Work out the finished part from the listing and answer in its coordinate system (mm). A direction names the side the tool comes from. Coordinates: 2 decimals unless noted, no trailing zeros. Loops run counter-clockwise (first coordinate to the right, second up) from the corner with the lowest first, then second, coordinate; pieces in that order, holes last. Notation, with made-up numbers: (0, 15.5) -> (26, 15.5) arc R7 cw to (26, 23.5) -> close; hole circle Ø4 at (67.5, 63.25). An arc over 180 degrees is marked (long way). Answer as CSV lines item,"result".
```python
from build123d import *

# Parameters (mm, degrees)
PAD_DEPTH         = 2
PAD001_DEPTH      = 4
PAD002_DEPTH      = 8
SKETCH002_R       = 2.5
PAD003_DEPTH      = 22.4
CYLINDER_R        = 6
CYLINDER_DEPTH    = 4
CYLINDER001_R     = 6
CYLINDER001_DEPTH = 4
CYLINDER002_R     = 6
CYLINDER002_DEPTH = 4
CYLINDER003_R     = 6
CYLINDER003_DEPTH = 4
CYLINDER004_R     = 3
CYLINDER004_DEPTH = 2
CYLINDER005_R     = 3
CYLINDER005_DEPTH = 2
CYLINDER006_R     = 3
CYLINDER006_DEPTH = 2
CYLINDER007_R     = 3
CYLINDER007_DEPTH = 2
SKETCH003_R       = 1.65
POCKET_DEPTH      = 22.4


with BuildPart() as part:
    # Sketch004 → Pad (new body)
    with BuildSketch(Plane.XY):
        with BuildLine():
            Line((74.149994, 7), (74.149994, 114.650046))
            ThreePointArc((74.149994, 114.650046), (72.099741, 119.599793), (67.149994, 121.650046))
            Line((67.149994, 121.650046), (7, 121.650046))
            ThreePointArc((7, 121.650046), (2.050253, 119.599793), (0, 114.650046))
            Line((0, 114.650046), (0, 7))
            ThreePointArc((0, 7), (2.050253, 2.050253), (7, 0))
            Line((7, 0), (67.149994, 0))
            ThreePointArc((67.149994, 0), (72.099741, 2.050253), (74.149994, 7))
        make_face()
    extrude(amount=PAD_DEPTH)

    # Sketch001 → Pad001 (join)
    with BuildSketch(Plane.XY):
        with BuildLine():
            Line((74.149994, 7), (74.149994, 114.650046))
            ThreePointArc((74.149994, 114.650046), (72.099741, 119.599793), (67.149994, 121.650046))
            Line((67.149994, 121.650046), (7, 121.650046))
            ThreePointArc((7, 121.650046), (2.050253, 119.599793), (0, 114.650046))
            Line((0, 114.650046), (0, 7))
            ThreePointArc((0, 7), (2.050253, 2.050253), (7, 0))
            Line((7, 0), (67.149994, 0))
            ThreePointArc((67.149994, 0), (72.099741, 2.050253), (74.149994, 7))
        make_face()
        with BuildLine():
            Line((7, 3), (67.149994, 3))
            ThreePointArc((67.149994, 3), (69.978421, 4.171573), (71.149994, 7))
            Line((71.149994, 7), (71.149994, 114.650046))
            ThreePointArc((71.149994, 114.650046), (69.978421, 117.478473), (67.149994, 118.650046))
            Line((67.149994, 118.650046), (7, 118.650046))
            ThreePointArc((7, 118.650046), (4.171573, 117.478473), (3, 114.650046))
            Line((3, 114.650046), (3, 7))
            ThreePointArc((3, 7), (4.171573, 4.171573), (7, 3))
        make_face(mode=Mode.SUBTRACT)
    extrude(amount=PAD001_DEPTH)

    # Sketch → Pad002 (join)
    with BuildSketch(Plane.XY):
        with BuildLine():
            Line((74.149994, 7), (74.149994, 114.650046))
            ThreePointArc((74.149994, 114.650046), (72.099741, 119.599793), (67.149994, 121.650046))
            Line((67.149994, 121.650046), (7, 121.650046))
            ThreePointArc((7, 121.650046), (2.050253, 119.599793), (0, 114.650046))
            Line((0, 114.650046), (0, 7))
            ThreePointArc((0, 7), (2.050253, 2.050253), (7, 0))
            Line((7, 0), (67.149994, 0))
            ThreePointArc((67.149994, 0), (72.099741, 2.050253), (74.149994, 7))
        make_face()
        with BuildLine():
            Line((7, 1.4), (67.149994, 1.4))
            ThreePointArc((67.149994, 1.4), (71.109792, 3.040202), (72.749994, 7))
            Line((72.749994, 7), (72.749994, 114.650046))
            ThreePointArc((72.749994, 114.650046), (71.109792, 118.609844), (67.149994, 120.250046))
            Line((67.149994, 120.250046), (7, 120.250046))
            ThreePointArc((7, 120.250046), (3.040202, 118.609844), (1.4, 114.650046))
            Line((1.4, 114.650046), (1.4, 7))
            ThreePointArc((1.4, 7), (3.040202, 3.040202), (7, 1.4))
        make_face(mode=Mode.SUBTRACT)
    extrude(amount=PAD002_DEPTH)

    # Sketch002 → Pad003 (join)
    with BuildSketch(Plane.XY):
        with Locations((12.075062, 22.075062)):
            Circle(SKETCH002_R)
        with Locations((12.075024, 109.57503)):
            Circle(SKETCH002_R)
        with Locations((62.075044, 109.575056)):
            Circle(SKETCH002_R)
        with Locations((62.075039, 22.075116)):
            Circle(SKETCH002_R)
    extrude(amount=PAD003_DEPTH)

    # Cylinder → Cylinder (join)
    with BuildSketch(Plane(origin=(12.075062, 22.075062, 0), x_dir=(0, -1, 0), z_dir=(0, 0, 1))):
        Circle(CYLINDER_R)
    extrude(amount=CYLINDER_DEPTH)

    # Cylinder001 → Cylinder001 (join)
    with BuildSketch(Plane(origin=(62.075039, 22.075116, 0), x_dir=(0, -1, 0), z_dir=(0, 0, 1))):
        Circle(CYLINDER001_R)
    extrude(amount=CYLINDER001_DEPTH)

    # Cylinder002 → Cylinder002 (join)
    with BuildSketch(Plane(origin=(62.075044, 109.575056, 0), x_dir=(0, -1, 0), z_dir=(0, 0, 1))):
        Circle(CYLINDER002_R)
    extrude(amount=CYLINDER002_DEPTH)

    # Cylinder003 → Cylinder003 (join)
    with BuildSketch(Plane(origin=(12.075024, 109.57503, 0), x_dir=(0, -1, 0), z_dir=(0, 0, 1))):
        Circle(CYLINDER003_R)
    extrude(amount=CYLINDER003_DEPTH)

    # Cylinder004 → Cylinder004 (cut)
    with BuildSketch(Plane(origin=(12.075062, 22.075062, 0), x_dir=(0, -1, 0), z_dir=(0, 0, 1))):
        Circle(CYLINDER004_R)
    extrude(amount=CYLINDER004_DEPTH, mode=Mode.SUBTRACT)

    # Cylinder005 → Cylinder005 (cut)
    with BuildSketch(Plane(origin=(62.075039, 22.075116, 0), x_dir=(0, -1, 0), z_dir=(0, 0, 1))):
        Circle(CYLINDER005_R)
    extrude(amount=CYLINDER005_DEPTH, mode=Mode.SUBTRACT)

    # Cylinder006 → Cylinder006 (cut)
    with BuildSketch(Plane(origin=(12.075024, 109.57503, 0), x_dir=(0, -1, 0), z_dir=(0, 0, 1))):
        Circle(CYLINDER006_R)
    extrude(amount=CYLINDER006_DEPTH, mode=Mode.SUBTRACT)

    # Cylinder007 → Cylinder007 (cut)
    with BuildSketch(Plane(origin=(62.075044, 109.575056, 0), x_dir=(0, -1, 0), z_dir=(0, 0, 1))):
        Circle(CYLINDER007_R)
    extrude(amount=CYLINDER007_DEPTH, mode=Mode.SUBTRACT)

    # Sketch003 → Pocket (cut)
    with BuildSketch(Plane.XY):
        with Locations((12.075062, 22.075062)):
            Circle(SKETCH003_R)
        with Locations((12.075024, 109.57503)):
            Circle(SKETCH003_R)
        with Locations((62.075044, 109.575056)):
            Circle(SKETCH003_R)
        with Locations((62.075039, 22.075116)):
            Circle(SKETCH003_R)
    extrude(amount=POCKET_DEPTH, mode=Mode.SUBTRACT)


solid = part.part
```
(1) Flat-ended cylindrical pins translate along their axes: pin 1 Ø5 at (x, y) = (13, 21) entering from -Z; pin 2 Ø6 at (x, z) = (17, 18.5) entering from -Y; pin 3 Ø10 at (x, z) = (45.5, 17) entering from +Y; pin 4 Ø6 at (x, y) = (14, 79.5) entering from +Z. Find the tip coordinate at first contact, or state that the pin passes through.
Computed values:
pin 1,"z = 0"
pin 2,"y = 20.48"
pin 3,"through"
pin 4,"z = 2"
(2) A cutting plane is placed at D-D, the plane y = 36. Write down the section's boundary in (x, z).
Computed values:
outline,"(0, 0) -> (74.15, 0) -> (74.15, 8) -> (72.75, 8) -> (72.75, 4) -> (71.15, 4) -> (71.15, 2) -> (3, 2) -> (3, 4) -> (1.4, 4) -> (1.4, 8) -> (0, 8) -> close"
(3) A cutting plane is placed at C-C, the plane x = 28. Write down the section's boundary in (y, z), and give its area (4 significant figures).
Computed values:
outline,"(0, 0) -> (121.65, 0) -> (121.65, 8) -> (120.25, 8) -> (120.25, 4) -> (118.65, 4) -> (118.65, 2) -> (3, 2) -> (3, 4) -> (1.4, 4) -> (1.4, 8) -> (0, 8) -> close"
area,"266.5 mm2"
(4) For a pull along Y with two mould halves and no side action, classify faces 1 (the face through (2, 2.1, 3.9)), 2 (the face through (11.717, 107.964, 12.057)), 3 (the face through (63, 108, 22.4)) as pulls with the +Y half, pulls with the -Y half, needs draft (parallel to the pull), parting line crosses it, or undercut.
Computed values:
face 1,"pulls with the -Y half"
face 2,"undercut"
face 3,"needs draft"
(5) A cutting plane is placed at B-B, the plane z = 5.75. Count the separate pieces of the cut face and the enclosed holes in it, and give its area (3 significant figures).
Computed values:
separate pieces,"5"
enclosed holes,"5"
area,"570 mm2"
(6) Which of the six approach directions +Z, -Z, +X, -X, +Y, -Y give full straight-line access (tool end or side, diameter ignored) to faces 4 (the face through (0, 62, 4)), 5 (the face through (61, 108, 2)), 6 (the face through (9.78, 16.53, 2.99))?
Computed values:
face 4,"+Z, -Z, -X, +Y, -Y"
face 5,"-Z"
face 6,"+Z"
(7) Consider line 1 along Y through (x, z) = (62, 7.5); line 2 along X through (y, z) = (70.5, 6); line 3 along Z through (x, y) = (57, 74). Determine where each line is inside the solid, lowest interval first.
Computed values:
line 1,"0 to 1.4, 19.58 to 20.43, 23.72 to 24.57, 107.08 to 107.93, 111.22 to 112.07, 120.25 to 121.65"
line 2,"0 to 1.4, 72.75 to 74.15"
line 3,"0 to 2"
(8) A cutting plane is placed at A-A, the plane z = 21. Write down the section's boundary in (x, y).
Computed values:
outline,"circle Ø5 at (12.08, 22.08); circle Ø5 at (12.08, 109.58); circle Ø5 at (62.08, 22.08); circle Ø5 at (62.08, 109.58); hole circle Ø3.3 at (12.08, 22.08); hole circle Ø3.3 at (12.08, 109.58); hole circle Ø3.3 at (62.08, 22.08); hole circle Ø3.3 at (62.08, 109.58)"
